Design review of the part built by this model. Coordinates are the model's own, in mm. Round coordinates to 2 decimals unless told otherwise and drop trailing zeros. Loops run counter-clockwise (first coordinate to the right, second up) from the corner with the lowest first, then second, coordinate; pieces in that order, holes last. Notation, with made-up numbers: (-15.5, 30) - (12.5, 30) arc R17 ccw to (12.5, 63) - close; hole circle Ø2 at (17.5, 8.25). An arc over 180 degrees is marked (long way). Use one line per item in the form item = value. Start each with the question number.
(1) For pin 1 (0.6 mm diameter, centred on x = 2, z = 1.5, fed in from -Y); pin 2 (3 mm diameter, centred on x = 3.3, y = 22.3, fed in from +Z); pin 3 (6.5 mm diameter, centred on x = 22.15, y = -14.7, fed in from -Z), all flat-tipped, find the tip position at first contact; note any pin that passes through.
(2) We need section B-B, the plane z = 1.6. Write out the cut boundary in (x, y).
(3) Wall thickness on probe 1 along X at (y, z) = (-15, 1.8); probe 2 along X at (y, z) = (6.5, 1.6); probe 3 along X at (y, z) = (-3, 1.2): over which ranges is each line inside the solid? List them lowest first. Write a range as [from, to].
(4) We need section C-C, the plane y = -10.5. Write out the cut boundary in (x, z).
(5) We need section A-A, the plane x = 20.5. Write out the cut boundary in (y, z).
(6) We need section D-D, the plane x = -5.5. Write out the cut boundary in (y, z), then the cut area to 3 significant figures.
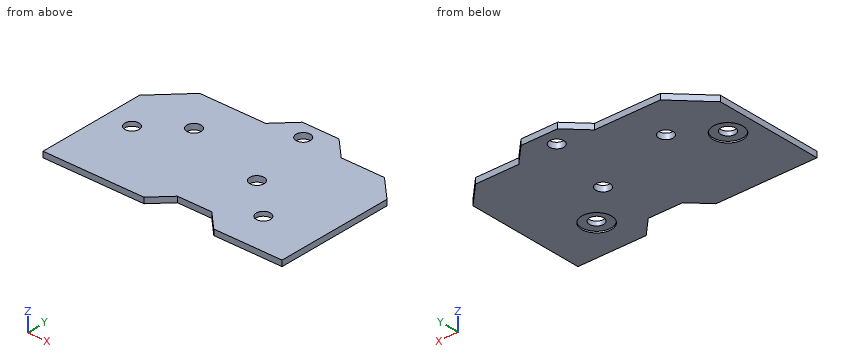
from build123d import *

# Parameters (mm, degrees)
SKETCH_1_R      = 5.2
SKETCH_1_R_2    = 2.5
EXTRUDE_1_DEPTH = 2
EXTRUDE_START   = -1.5
SKETCH_3_R      = 5.2
SKETCH_3_R_2    = 2.5
EXTRUDE_3_DEPTH = 1.5


with BuildPart() as part:
    # 스케치1 → 보스-돌출1 (new body)
    with BuildSketch(Plane.XY):
        Polygon((17.655171042, 21.115026673), (32.779698935, 21.115026673), (40.649680384, 13.245045225), (40.649680384, -28.196867314), (16.748789391, -28.196867314), (10.556633431, -22.004711354), (-1.494033315, -22.004711354), (-7.686189276, -28.196867314), (-43.049187557, -28.196867314), (-43.049187557, 9.964172757), (-31.898333641, 21.115026673), (-8.845568875, 21.115026673), (-2.011604239, 27.94899131), (10.821206405, 27.94899131), align=None)
        with Locations((22.149680384, -14.696867314)):
            Circle(SKETCH_1_R, mode=Mode.SUBTRACT)
        with Locations((-34.049187557, -3.196867314)):
            Circle(SKETCH_1_R, mode=Mode.SUBTRACT)
        with Locations((8.800246413, -2.196867314)):
            Circle(SKETCH_1_R_2, mode=Mode.SUBTRACT)
        with Locations((3.300246413, 22.303132686)):
            Circle(SKETCH_1_R_2, mode=Mode.SUBTRACT)
        with Locations((-21.199753587, 6.803132686)):
            Circle(SKETCH_1_R_2, mode=Mode.SUBTRACT)
    extrude(amount=EXTRUDE_1_DEPTH)

    # 스케치3 → 보스-돌출3 (add)
    # profile 1 of 2: a face of its own
    with BuildSketch(Plane.XY.offset(2).offset(EXTRUDE_START)):
        with Locations((-34.049187557, -3.196867314)):
            Circle(SKETCH_3_R)
        with Locations((-34.049187557, -3.196867314)):
            Circle(SKETCH_3_R_2, mode=Mode.SUBTRACT)
    # profile 2 of 2: a face of its own
    with BuildSketch(Plane.XY.offset(2).offset(EXTRUDE_START)):
        with Locations((22.149680384, -14.696867314)):
            Circle(SKETCH_3_R)
        with Locations((22.149680384, -14.696867314)):
            Circle(SKETCH_3_R_2, mode=Mode.SUBTRACT)
    extrude(amount=EXTRUDE_3_DEPTH)


solid = part.part
Data:
q1.pin_1 = -22
q1.pin_2 = through
q1.pin_3 = 0.5
q2.outline = (-43.05, -28.2) - (-7.69, -28.2) - (-1.49, -22) - (10.56, -22) - (16.75, -28.2) - (40.65, -28.2) - (40.65, 13.25) - (32.78, 21.12) - (17.66, 21.12) - (10.82, 27.95) - (-2.01, 27.95) - (-8.85, 21.12) - (-31.9, 21.12) - (-43.05, 9.96) - close; hole circle Ø5 at (-34.05, -3.2); hole circle Ø5 at (-21.2, 6.8); hole circle Ø5 at (3.3, 22.3); hole circle Ø5 at (8.8, -2.2); hole circle Ø5 at (22.15, -14.7)
q3.probe_1 = [-43.05, 19.67], [24.63, 40.65]
q3.probe_2 = [-43.05, -23.68], [-18.72, 40.65]
q3.probe_3 = [-43.05, -36.54], [-31.56, 6.43], [11.17, 40.65]
q4.outline = (-43.05, 0) - (19.08, 0) - (19.08, 0.5) - (25.22, 0.5) - (25.22, 0) - (40.65, 0) - (40.65, 2) - (-43.05, 2) - close
q5.outline = (-28.2, 0) - (-19.63, 0) - (-19.63, 0.5) - (-16.58, 0.5) - (-16.58, 2) - (-28.2, 2) - close; (-12.82, 0.5) - (-9.77, 0.5) - (-9.77, 0) - (21.12, 0) - (21.12, 2) - (-12.82, 2) - close
q6.outline = (-26.01, 0) - (24.46, 0) - (24.46, 2) - (-26.01, 2) - close
q6.area = 101 mm^2
